Autodesk Fusion 360 part; units mm, degrees
sketch "Sketch1" plane through (0, 0, 0) normal (0, 1, 0) x (1, 0, 0)
  circle A0 centre (0, 0) radius 3.8
  circle A1 centre (0, 0) radius 4.9
  circle A2 centre (0, 0) radius 2.85
  circle A3 centre (0, 0) radius 3.15
  dimension "d1" = 7.6
  dimension "d2" = 9.8
  dimension "d3" = 5.7
  dimension "d4" = 6.3
extrude "Extrude1" add sketch "Sketch1" against normal blind 10 contours A0 | A3
extrude "Extrude2" add sketch "Sketch1" along normal blind 10 contours A0 | A1
chamfer "Chamfer1" distance 0.5 angle 45 1 edges at (-3.5428, 0, 1.3741)
chamfer "Chamfer2" distance 0.3 angle 45 1 edges at (-2.6571, 0, -1.0306)
chamfer "Chamfer3" distance 0.5 angle 45 2 edges at (-2.6571, -10, 1.0306) (-2.9368, 10, -1.1391)
chamfer "Chamfer4" distance 0.5 angle 45 1 edges at (-4.5684, 0, 1.7719)
Build history of the part. All positions in model axes, mm. A direction names the side the tool comes from. Coordinates: 2 decimals unless noted, no trailing zeros. Write each loop counter-clockwise with the first axis right and the second up, starting at its lowest first coordinate (ties: lowest second). Pieces come first, ordered by that corner, then holes.
1. Drill centre lines: probe 1 along Z at (x, y) = (0, -3); probe 2 along X at (y, z) = (4, 0). Where is each one in solid material? Low to high.
Answer block:
probe 1: z = -3.8 to -2.85, 2.85 to 3.8
probe 2: x = -4.9 to -3.15, 3.15 to 4.9
2. Band-saw the part on C-C, the plane y = 3.5. Give the cut face in (x, z).
Answer block:
outline: circle Ø9.8 at (0, 0); hole circle Ø6.3 at (0, 0)
3. Band-saw the part on D-D, the plane y = -7.25. Give the cut face in (x, z).
Answer block:
outline: circle Ø7.6 at (0, 0); hole circle Ø5.7 at (0, 0)
4. Drop flat-ended pins along their axis: pin 1 (1.5 mm diameter, centred on x = 1.5, z = 0.5, fed in from +Y); pin 2 (4 mm diameter, centred on y = 5.5, z = -3, fed in from -X); pin 3 (1 mm diameter, centred on x = 3, y = 3.5, fed in from -Z); pin 4 (3 mm diameter, centred on y = 7, z = -2.5, fed in from +X). Give the stop position or say it passes through.
Answer block:
pin 1: passes through
pin 2: stops at x = -4.8
pin 3: stops at z = -4.21
pin 4: stops at x = 4.8
5. Pull direction X, two halves, no side cores. Call faces 3 (the cylindrical face through (-1.062, 5.184, -4.783)), 4 (the cylindrical face through (-2.5, 4.684, -1.917)), 5 (the flat face through (0, 10, -4)): released by +X, released by -X, zero draft, split by the parting line, or undercut.
Answer block:
face 3: split by the parting line
face 4: undercut
face 5: zero draft
6. 3-axis set-ups, long thin cutter, end or side, ignore diameter. For faces 1 (the flat face through (2, -10, 3)), 2 (the cylindrical face through (-3.796, -5.184, -0.167)): which of +Z, -Z, +X, -X, +Y, -Y reach the whole face in a straight line?
Answer block:
face 1: +Z, -Z, +X, -X, -Y
face 2: -Y
